Part model, mm, in its own coordinate system. A direction names the side the tool comes from. Give positions to 0.01 mm unless a question says otherwise; leave off trailing zeros. Loops run counter-clockwise (first coordinate to the right, second up) from the corner with the lowest first, then second, coordinate; pieces in that order, holes last. Notation, with made-up numbers: M -17,-9 L 9,-9 A27 cw 9,9 Z; hole C -20.75,-1.75 d10. An arc over 180 degrees is marked long. Answer in a Markdown table with one row per item.
from build123d import *

# Parameters (mm, degrees)
SCHIZZO14_R                  = 10
ESTRUSIONE_ESTRUSIONE2_DEPTH = 2
FORO_3_0_3_1_D               = 3
SCHIZZO19_R                  = 4.5
ESTRUSIONE_ESTRUSIONE3_DEPTH = 2
SCHIZZO20_R                  = 1.625
TAGLIO_ESTRUSIONE1_DEPTH     = 5


with BuildPart() as part:
    # Schizzo14 → Estrusione-Estrusione2 (new body)
    with BuildSketch(Plane.XY):
        Circle(SCHIZZO14_R)
    extrude(amount=ESTRUSIONE_ESTRUSIONE2_DEPTH)

    # Foro Ø3.0 (3)-1 (through all)
    with Locations(Plane(origin=(7.13, 0, 0), x_dir=(-1, 0, 0), z_dir=(0, 0, -1))):
        with Locations((0, 0), (14.26, 0), (7.13, -7.13), (7.13, 7.13)):
            Hole(FORO_3_0_3_1_D / 2)

    # Schizzo19 → Estrusione-Estrusione3 (add)
    with BuildSketch(Plane.XY):
        Circle(SCHIZZO19_R)
    extrude(amount=-ESTRUSIONE_ESTRUSIONE3_DEPTH)

    # Schizzo20 → Taglio-Estrusione1 (cut, through all)
    with BuildSketch(Plane(origin=(0, 0, -2), x_dir=(-1, 0, 0), z_dir=(0, 0, -1))):
        Circle(SCHIZZO20_R)
    extrude(amount=-TAGLIO_ESTRUSIONE1_DEPTH, mode=Mode.SUBTRACT)


solid = part.part
(1) Drill centre lines: line 1 along Y through (x, z) = (0, 1.55) (3 decimals); line 2 along Y through (x, z) = (-1.25, 0.2); line 3 along Y through (x, z) = (0, -0.3) (3 decimals). Where is each one in solid material? Low to high.
Recorded:
| item | result |
|---|---|
| line 1 | y = -10 to -8.63, -5.63 to -1.625, 1.625 to 5.63, 8.63 to 10 |
| line 2 | y = -9.92 to -7.96, -6.3 to -1.04, 1.04 to 6.3, 7.96 to 9.92 |
| line 3 | y = -4.5 to -1.625, 1.625 to 4.5 |
(2) Saw through at C-C (x = -6.25). Write the cut outline in (y, z).
Recorded:
| item | result |
|---|---|
| outline | M -7.81,0 L -1.21,0 L -1.21,2 L -7.81,2 Z; M 1.21,0 L 7.81,0 L 7.81,2 L 1.21,2 Z |
(3) Saw through at A-A (y = 0). Write the cut outline in (x, z) (3 decimals), plus the area to 3 significant figures.
Recorded:
| item | result |
|---|---|
| outline | M -10,0 L -8.63,0 L -8.63,2 L -10,2 Z; M -5.63,0 L -4.5,0 L -4.5,-2 L -1.625,-2 L -1.625,2 L -5.63,2 Z; M 1.625,-2 L 4.5,-2 L 4.5,0 L 5.63,0 L 5.63,2 L 1.625,2 Z; M 8.63,0 L 10,0 L 10,2 L 8.63,2 Z |
| area | 33.0 mm^2 |
(4) Which spindle directions (+Z, -Z, +X, -X, +Y, -Y) get a long thin tool onto all of the face, cutting with end or side? Do faces 1 (the face through (4.3, -2.1, 0)), 2 (the face through (-0.3, -8.6, 1)). Say none if no direction does.
Recorded:
| item | result |
|---|---|
| face 1 | -Z |
| face 2 | +Z, -Z |
(5) Saw through at B-B (z = 1.7). Write the cut outline in (x, y) (3 decimals), plus the area to 3 significant figures.
Recorded:
| item | result |
|---|---|
| outline | C 0,0 d20; hole C -7.13,0 d3; hole C 0,0 d3.25; hole C 0,-7.13 d3; hole C 0,7.13 d3; hole C 7.13,0 d3 |
| area | 278 mm^2 |
(6) Pin check, flat tips, straight feed: pin 1 Ø1 at (x, z) = (1, 0) entering from -Y; pin 2 Ø2.5 at (x, y) = (0, -7.13) entering from +Z; pin 3 Ø12 at (x, y) = (7, 0) entering from -Z; pin 4 Ø5 at (x, y) = (0, 7.13) entering from -Z. Stop position of each tip, or through.
Recorded:
| item | result |
|---|---|
| pin 1 | stops at y = -9.99 |
| pin 2 | passes through |
| pin 3 | stops at z = -2 |
| pin 4 | stops at z = 0 |
(7) Pull direction Y, two halves, no side cores. Call faces 3 (the face through (-2.17, -9.76, 0.99)), 4 (the face through (0, -2, 2)), 5 (the face through (-0.325, 5.666, 1.014)): +Y half, -Y half, draft (parallel to the pull), parting line (faces both ways), or undercut.
Recorded:
| item | result |
|---|---|
| face 3 | parting line |
| face 4 | draft |
| face 5 | undercut |
